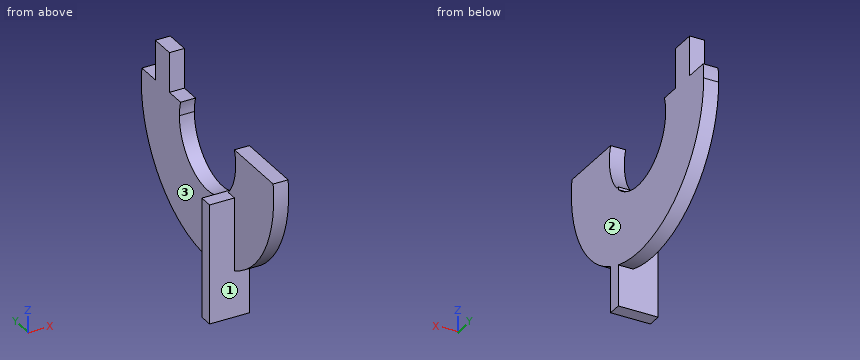
from build123d import *

# Parameters (mm, degrees)
F3_W          = 5
F3_H          = 8
F4_DEPTH      = 3
F5_DEPTH      = 5
F5_DEPTH_BACK = 3


with BuildPart() as f4:
    # F3 (on Right) → F4 (new body)
    with BuildSketch(Plane.YZ):
        with BuildLine():
            ThreePointArc((19.1383222897, 0.0889776102), (19.469019625, -1.3642024736), (19.5800742792, -2.8503922149))
            ThreePointArc((19.5800742792, -2.8503922149), (13.5612334827, -12.023743369), (2.75, -10.1545064899))
            Line((2.75, -10.1545064899), (2.75, -25.3359450287))
            ThreePointArc((2.75, -25.3359450287), (23.5754887861, -21.7283786748), (33.0800742792, -2.8503922149))
            ThreePointArc((33.0800742792, -2.8503922149), (33.0338908423, -1.3778133128), (32.8955220559, 0.0889776102))
            Line((32.8955220559, 0.0889776102), (28.1147146076, 0.0889776102))
            Line((28.1147146076, 0.0889776102), (23.1147146076, 0.0889776102))
            Line((23.1147146076, 0.0889776102), (19.1383222897, 0.0889776102))
        make_face()
        with BuildLine():
            ThreePointArc((2.2018949322, -9.6003899574), (-0.1760316999, -5.0454767522), (0.0218262686, 0.0889776102))
            Line((0.0218262686, 0.0889776102), (-13.7353734976, 0.0889776102))
            ThreePointArc((-13.7353734976, 0.0889776102), (-10.8978226866, -14.3788672164), (0, -24.3090076597))
            Line((0, -24.3090076597), (0, -9.6003899574))
            Line((0, -9.6003899574), (2.2018949322, -9.6003899574))
        make_face()
        with BuildLine():
            Line((2.75, -25.3359450287), (2.75, -10.1545064899))
            ThreePointArc((2.75, -10.1545064899), (2.4705469349, -9.8827901659), (2.2018949322, -9.6003899574))
            Line((2.2018949322, -9.6003899574), (0, -9.6003899574))
            Line((0, -9.6003899574), (0, -24.3090076597))
            ThreePointArc((0, -24.3090076597), (1.3589494159, -24.8654576471), (2.75, -25.3359450287))
        make_face()
        with Locations((25.6147146076, 4.0889776102)):
            Rectangle(F3_W, F3_H)
    extrude(amount=F4_DEPTH)

    # F3 (on Right) → F5 (join, two sides)
    with BuildSketch(Plane.YZ) as f5_sk:
        with BuildLine():
            ThreePointArc((2.2018949322, -9.6003899574), (2.4705469349, -9.8827901659), (2.75, -10.1545064899))
            Line((2.75, -10.1545064899), (2.75, -9.6003899574))
            Line((2.75, -9.6003899574), (2.2018949322, -9.6003899574))
        make_face()
        with BuildLine():
            Line((2.75, -25.3359450287), (2.75, -10.1545064899))
            ThreePointArc((2.75, -10.1545064899), (2.4705469349, -9.8827901659), (2.2018949322, -9.6003899574))
            Line((2.2018949322, -9.6003899574), (0, -9.6003899574))
            Line((0, -9.6003899574), (0, -24.3090076597))
            ThreePointArc((0, -24.3090076597), (1.3589494159, -24.8654576471), (2.75, -25.3359450287))
        make_face()
        with BuildLine():
            Line((2.75, -33.6003899574), (2.75, -25.3359450287))
            ThreePointArc((2.75, -25.3359450287), (1.3589494159, -24.8654576471), (0, -24.3090076597))
            Line((0, -24.3090076597), (0, -33.6003899574))
            Line((0, -33.6003899574), (2.75, -33.6003899574))
        make_face()
    extrude(amount=-F5_DEPTH)
    extrude(f5_sk.sketch, amount=F5_DEPTH_BACK)


solid = f4.part
For this review, take the finished solid that the model builds, in its own axes (mm). Face numbers are marked on the shaded views. A direction names the side the tool comes from. Coordinates: 2 decimals unless noted, no trailing zeros. Order: outer loops, then holes, each group sorted by start corner. A loop starts at its lowest first (then second) coordinate and runs counter-clockwise, first axis right, second up. Notation, with made-up numbers: (43, -13) -> (97, -13) arc R19 ccw to (97, -8) -> close; hole circle Ø9 at (-30.75, 50.25). An arc over 180 degrees is marked (long way). Return JSON: item names as keys, results as strings.
1. For line 1 (Y direction, x = 1.5, z = -3); line 2 (X direction, y = 17.5, z = -18); line 3 (Y direction, x = -1, z = -21), list the stretches that pass through material, from the lowest coordinate up. Write a range as from..to.
Answer block:
{"line 1": "-13.92..-0.42, 19.58..33.08", "line 2": "0..3", "line 3": "0..2.75"}
2. We need section C-C on y = 24. Write out the cut boundary in (x, z), and give its area (3 significant figures).
Answer block:
{"outline": "(0, -21.41) -> (3, -21.41) -> (3, 8.09) -> (0, 8.09) -> close", "area": "88.5 mm²"}
3. We need section B-B on x = -3. Write out the cut boundary in (y, z), and give its area (3 significant figures).
Answer block:
{"outline": "(0, -33.6) -> (2.75, -33.6) -> (2.75, -9.6) -> (0, -9.6) -> close", "area": "66.0 mm²"}
4. Machinability: for the marked faces 1, 2 and 3, which of the approach directions +Z, -Z, +X, -X, +Y, -Y give a long, thin tool a straight path to every point of the face, cutting with its end or side? Answer none if there is none.
Answer block:
{"face 1": "-Z, -X, -Y", "face 2": "+Z, -Z, +X, +Y, -Y", "face 3": "+Z, -Z, -X, +Y"}
5. We need section A-A on z = -5.5. Write out the cut boundary in (x, y).
Answer block:
{"outline": "(0, -13.77) -> (3, -13.77) -> (3, -0.06) -> (0, -0.06) -> close; (0, 19.22) -> (3, 19.22) -> (3, 32.93) -> (0, 32.93) -> close"}
6. For pin 1 Ø2 at (x, y) = (-2.5, 1.5) entering from +Z; pin 2 Ø2.5 at (x, y) = (1, 29.5) entering from +Z; pin 3 Ø3.5 at (x, z) = (1, 5) entering from +Y; pin 4 Ø3 at (y, z) = (-4, 2) entering from -X, all flat-tipped, find the tip position at first contact; note any pin that passes through.
Answer block:
{"pin 1": "z = -9.6", "pin 2": "z = 0.09", "pin 3": "y = 28.11", "pin 4": "through"}
7. We need section D-D on x = 1.25. Write out the cut boundary in (y, z), and give its area (3 significant figures).
Answer block:
{"outline": "(-13.74, 0.09) arc R23.5 ccw to (0, -24.31) -> (0, -33.6) -> (2.75, -33.6) -> (2.75, -25.34) arc R23.5 ccw to (32.9, 0.09) -> (28.11, 0.09) -> (28.11, 8.09) -> (23.11, 8.09) -> (23.11, 0.09) -> (19.14, 0.09) arc R10 cw to (2.75, -10.15) -> (2.75, -9.6) -> (2.2, -9.6) arc R10 cw to (0.02, 0.09) -> close", "area": "854 mm²"}
